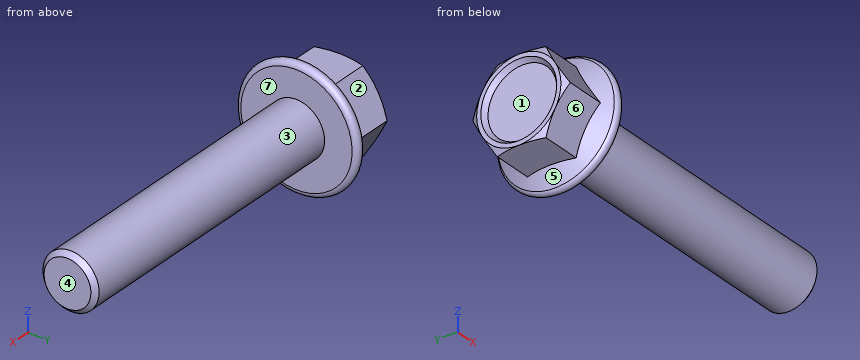
```python
from build123d import *

# Parameters (mm, degrees)
SKETCH2_R           = 4.7625
BOSS_EXTRUDE1_DEPTH = 50.8
CHAMFER1_SIZE       = 0.793750063
BOSS_EXTRUDE2_DEPTH = 9.921875
SKETCH5_OUTSIDE_W   = 70.482
SKETCH5_OUTSIDE_H   = 70.482
SKETCH5_OUTSIDE_R   = 7.14375
CUT_EXTRUDE1_DEPTH  = 9.921875
CUT_EXTRUDE1_DRAFT  = -60
SKETCH6_R           = 6.429375
CUT_EXTRUDE2_DEPTH  = 0.826822917
CUT_EXTRUDE2_DRAFT  = -35
SKETCH14_W          = 25.4
SKETCH14_H          = 4.7625


with BuildPart() as part:
    # Sketch2 → Boss-Extrude1 (new body)
    with BuildSketch(Plane(origin=(0, 0, 0), x_dir=(0, 0, -1), z_dir=(1, 0, 0))):
        Circle(SKETCH2_R)
    extrude(amount=BOSS_EXTRUDE1_DEPTH)

    # Chamfer1
    chamfer1_edges = [part.edges().sort_by_distance(p)[0] for p in [
        (50.8, 0, 4.7625),
    ]]
    chamfer(chamfer1_edges, length=CHAMFER1_SIZE)

    # Sketch3 → Boss-Extrude2 (add)
    with BuildSketch(Plane.ZY):
        Polygon((0, 8.248891971), (-7.14375, 4.124445986), (-7.14375, -4.124445986), (0, -8.248891971), (7.14375, -4.124445986), (7.14375, 4.124445986), align=None)
    extrude(amount=BOSS_EXTRUDE2_DEPTH)

    # Sketch4 → Revolve1 (revolve)
    with BuildSketch(Plane.XY, mode=Mode.PRIVATE) as revolve1_sk:
        with BuildLine():
            Line((0, 0), (0, 9.432563869))
            ThreePointArc((0, 9.432563869), (-0.656824283, 10.28855394), (-1.653645833, 9.875656934))
            Line((-1.653645833, 9.875656934), (-3.230913037, 7.14375))
            Line((-3.230913037, 7.14375), (-3.230913037, 0))
            Line((-3.230913037, 0), (0, 0))
        make_face()
    revolve(revolve1_sk.sketch.rotate(Axis((-3.230913037, 0, 0), (1, 0, 0)), 180), axis=Axis((-3.230913037, 0, 0), (1, 0, 0)))


with BuildPart() as cut_extrude1_tool:
    # Sketch5 outside → Cut-Extrude1 (with draft: the straight prism first)
    with BuildSketch(Plane.ZY.offset(9.921875)):
        Rectangle(SKETCH5_OUTSIDE_W, SKETCH5_OUTSIDE_H)
        Circle(SKETCH5_OUTSIDE_R, mode=Mode.SUBTRACT)
    extrude(amount=-CUT_EXTRUDE1_DEPTH)
    # Cut-Extrude1: the draft: its side faces are tilted about the plane it starts from
    cut_extrude1_sides = [cut_extrude1_tool.faces().sort_by_distance(p)[0] for p in [
        (-4.9609375, -35.241, 0),
        (-4.9609375, 0, 35.241),
        (-4.9609375, 35.241, 0),
        (-4.9609375, 0, -35.241),
        (-4.9609375, 0, -7.14375),
    ]]
    draft(cut_extrude1_sides, Plane.ZY.offset(9.921875), CUT_EXTRUDE1_DRAFT)


with BuildPart() as part_1:
    add(part.part)

    # Cut-Extrude1: cut by cut_extrude1_tool
    add(cut_extrude1_tool.part, mode=Mode.SUBTRACT)


with BuildPart() as cut_extrude2_tool:
    # Sketch6 → Cut-Extrude2 (with draft: the straight prism first)
    with BuildSketch(Plane.ZY.offset(9.921875)):
        Circle(SKETCH6_R)
    extrude(amount=-CUT_EXTRUDE2_DEPTH)
    # Cut-Extrude2: the draft: its side faces are tilted about the plane it starts from
    cut_extrude2_sides = [cut_extrude2_tool.faces().sort_by_distance(p)[0] for p in [
        (-9.508463542, 0, -6.429375),
    ]]
    draft(cut_extrude2_sides, Plane.ZY.offset(9.921875), CUT_EXTRUDE2_DRAFT)


with BuildPart() as part_2:
    add(part_1.part)

    # Cut-Extrude2: cut by cut_extrude2_tool
    add(cut_extrude2_tool.part, mode=Mode.SUBTRACT)

    # Sketch14 → Revolve2 (revolve)
    with BuildSketch(Plane.XY, mode=Mode.PRIVATE) as revolve2_sk:
        with Locations((12.7, 2.38125)):
            Rectangle(SKETCH14_W, SKETCH14_H)
    revolve(revolve2_sk.sketch.rotate(Axis((0, 0, 0), (1, 0, 0)), 90), axis=Axis((0, 0, 0), (1, 0, 0)))


solid = part_2.part
```
The listing builds one solid part. Answer for the finished solid, in the listing's coordinates (mm). Face numbers are marked on the shaded views. A direction names the side the tool comes from. Round coordinates to 2 decimals unless told otherwise and drop trailing zeros. Write each loop counter-clockwise with the first axis right and the second up, starting at its lowest first coordinate (ties: lowest second). Pieces come first, ordered by that corner, then holes. Notation, with made-up numbers: (23, -3) -> (65, -3) arc R35 ccw to (65, 36) -> close; hole circle Ø7 at (17, -30). An arc over 180 degrees is marked (long way). Answer as a JSON object with one key per item and string values. Group by question number.
Q1. Section B-B (x = -1) is taken. Write down the section's boundary in (y, z), plus the area to 3 significant figures.
Q2. Section A-A (x = 39.5) is taken. Write down the section's boundary in (y, z) (1 decimal).
Q3. Which of the six approach directions +Z, -Z, +X, -X, +Y, -Y give full straight-line access (tool end or side, diameter ignored) to the marked faces 5, 6 and 7?
Q4. Each of these flat-tipped pins is pushed along its axis until it touches: pin 1 Ø1.5 at (x, y) = (5, 3) entering from +Z; pin 2 Ø8 at (x, z) = (36, -0.5) entering from +Y; pin 3 Ø8 at (x, z) = (34.5, -7.5) entering from +Y; pin 4 Ø6 at (y, z) = (1, 4) entering from -X. Where does it stop, or does it pass through?
Q5. Straight lines are drawn through the part: line 1 along X through (y, z) = (2.5, 1.75); line 2 along X through (y, z) = (4.75, -1.5); line 3 along Y through (x, z) = (42, -0.25). For each, find the intervals that lie inside material, in ascending order.
Q6. Determine the mould class of the marked faces 1, 2, 3 and 4 for opening direction Z: pulls with the +Z half, pulls with the -Z half, needs draft (parallel to the pull), parting line crosses it, or undercut.
Check values:
{
 "1": {"outline": "circle Ø20.62 at (0, 0)", "area": "334 mm^2"},
 "2": {"outline": "circle Ø9.5 at (0, 0)"},
 "3": {"face 5": "-X", "face 6": "-Z, -X, -Y", "face 7": "+X"},
 "4": {"pin 1": "z = 4.2", "pin 2": "y = 4.76", "pin 3": "y = 3.23", "pin 4": "x = -9.92"},
 "5": {"line 1": "-9.1 to 50.8", "line 2": "-9.1 to 0", "line 3": "-4.76 to 4.76"},
 "6": {"face 1": "undercut", "face 2": "pulls with the +Z half", "face 3": "parting line crosses it", "face 4": "needs draft"}
}
